Geometry check sheet. Reference: the model listing, model coordinates, mm. Face numbers are marked on the shaded views. Give positions to 0.01 mm unless a question says otherwise; leave off trailing zeros.
(1) Mould release check, pull along Z, two halves, no side actions. Record for the marked faces 1, 2 and 3: +Z half, -Z half, draft (parallel to the pull), parting line (faces both ways), or undercut.
(2) Thickness scan on line 1 along Z through (x, y) = (1.5, -2); line 2 along X through (y, z) = (0.25, -1); line 3 along X through (y, z) = (0.5, -0.75). Record the ranges inside material, lowest first.
(3) Depth check by flat-ended pin: P1, Ø1.2, axis at x = 0.5, y = 1, coming from the +Z side; P2, Ø2, axis at y = 1, z = 1, coming from the -X side; P3, Ø1.2, axis at x = 1, z = 1, coming from the -Y side; P4, Ø0.8, axis at x = 0.5, y = 1, coming from the -Z side. Enter the tip coordinate at first touch or a pass-through.
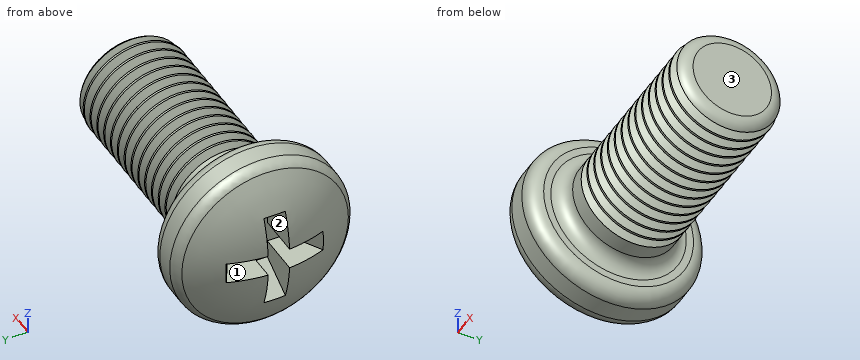
```python
from build123d import *

# Parameters (mm, degrees)
CUT_EXTRUDE1_DEPTH = 1.2
FILLET1_R          = 0.4
DRAFT1_ANGLE       = -30
LPATTERN10_COUNT   = 14
LPATTERN10_PITCH   = 0.36


with BuildPart() as part:
    # Sketch1 → Base (revolve)
    with BuildSketch(Plane.XY, mode=Mode.PRIVATE) as base_sk:
        with BuildLine():
            Line((8, 0), (8, 1.5))
            Line((8, 1.5), (2, 1.5))
            Line((2, 1.5), (2, 2.5))
            Line((2, 2.5), (0.877501001, 2.5))
            ThreePointArc((0.877501001, 2.5), (0.225745372, 1.324764885), (0, 0))
            Line((0, 0), (8, 0))
        make_face()
    revolve(base_sk.sketch.rotate(Axis((-8.635649275, 0, 0), (1, 0, 0)), 180), axis=Axis((-8.635649275, 0, 0), (1, 0, 0)))

    # Sketch2 → Cut-Extrude1 (cut)
    with BuildSketch(Plane(origin=(0, 0, 0), x_dir=(0, 0, -1), z_dir=(1, 0, 0))):
        Polygon((-0.3, 1.5), (0.3, 1.5), (0.3, 0.3), (1.5, 0.3), (1.5, -0.3), (0.3, -0.3), (0.3, -1.5), (-0.3, -1.5), (-0.3, -0.3), (-1.5, -0.3), (-1.5, 0.3), (-0.3, 0.3), align=None)
    extrude(amount=CUT_EXTRUDE1_DEPTH, mode=Mode.SUBTRACT)

    # Fillet1
    fillet1_edges = [part.edges().sort_by_distance(p)[0] for p in [
        (0.877501001, 2.5, 0),
        (2, 2.5, 0),
        (2, 1.5, 0),
        (8, 1.5, 0),
    ]]
    fillet(fillet1_edges, radius=FILLET1_R)

    # Draft1
    draft1_faces = [part.faces().sort_by_distance(p)[0] for p in [
        (0.747967708, 1.5, 0),
        (0.747967708, 0, 1.5),
        (0.747967708, -1.5, 0),
        (0.747967708, 0, -1.5),
    ]]
    draft(draft1_faces, Plane(origin=(0, 0, 0), x_dir=(0, 0, 1), z_dir=(1, 0, 0)), DRAFT1_ANGLE)

    # Sketch3 → Cut-Revolve10 (revolve, cut)
    with BuildSketch(Plane.XY, mode=Mode.PRIVATE) as cut_revolve10_sk:
        Polygon((2.85, 1.8), (3.15, 1.8), (3.15, 1.5), (3, 1.240192379), (2.85, 1.5), align=None)
    cut_revolve10 = revolve(cut_revolve10_sk.sketch.rotate(Axis((0, 0, 0), (1, 0, 0)), 90), axis=Axis((0, 0, 0), (1, 0, 0)), mode=Mode.SUBTRACT)

    # LPattern10: Cut-Revolve10 ×14
    with Locations(*[(i * LPATTERN10_PITCH, 0, 0) for i in range(1, LPATTERN10_COUNT)]):
        add(cut_revolve10, mode=Mode.SUBTRACT)


solid = part.part
```
Reply:
1. face 1: undercut
1. face 2: undercut
1. face 3: draft
2. line 1: z = -1.5 to 1.5
2. line 2: x = 0.87 to 8
2. line 3: x = 0.1 to 8
3. P1: stops at z = 2.41
3. P2: stops at x = 0.02
3. P3: stops at y = -2.47
3. P4: stops at z = -2.29
